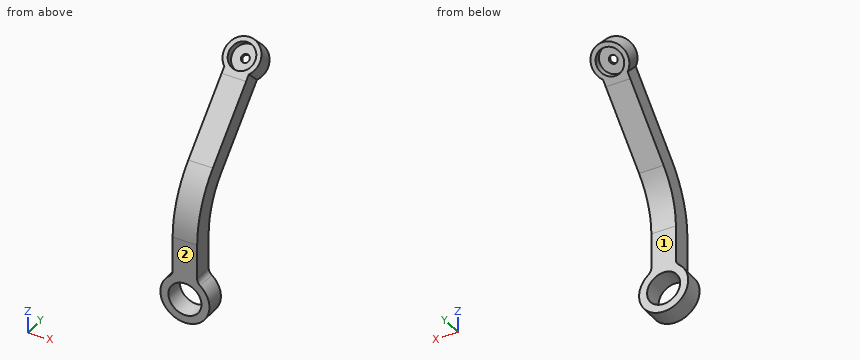
Autodesk Inventor part; units mm, degrees
ref_plane "Work Plane11" through (7.5, 8.6447, 72.635) normal (0, 0.7071, -0.7071) x (-1, 0, 0)
ref_plane "YZ Plane" through (0, 0, 0) normal (1, 0, 0) x (0, 1, 0)
ref_plane "XZ Plane" through (0, 0, 0) normal (0, 1, 0) x (-1, 0, 0)
sketch "Sketch1" plane through (0, 0, 0) normal (0, 1, 0) x (-1, 0, 0)
  arc A0 (-9.375, 11.7094) -> (9.375, 11.7094) centre (0, 0) ccw
  line L0 (-7.5, 15.6125) -> (-7.5, 22.9904)
  line L1 (7.5, 22.9904) -> (7.5, 15.6125)
  line L2 (7.5, 22.9904) -> (-7.5, 22.9904)
  arc A1 (7.5, 15.6125) -> (9.375, 11.7094) centre (12.5, 15.6125) ccw
  arc A2 (-9.375, 11.7094) -> (-7.5, 15.6125) centre (-12.5, 15.6125) ccw
  point P0 (7.5, 12.9904)
  point P1 (-7.5, 12.9904)
  point P2 (0, 12.9904)
  point P3 (0, 22.9904)
  dimension "d0" = 30
  dimension "d109" = 5
  dimension "d129" = 15
  dimension "d131" = 10
  dimension "d132" = 12.9904
extrude "Extrusion1" add sketch "Sketch1" against normal blind 12
sketch "Sketch22" plane through (-7.5, 0, 22.9904) normal (0, 0, 1) x (1, 0, 0)
  line L0 (0, 0) -> (0, -12)
  line L1 (15, -12) -> (0, -12)
  line L2 (0, 0) -> (15, 0)
  line L3 (15, 0) -> (15, -12)
  line L4 (15, -12) -> (0, -12)
  line L5 (0, -12) -> (0, 0)
  point P0 (7.5, 0)
sketch "Sketch23" plane through (0, 0, 0) normal (1, 0, 0) x (0, 1, 0)
  line L0 (0, 22.9904) -> (-12, 22.9904)
  line L1 (-6, 22.9904) -> (-6, 37.2797)
  line L2 (8.6447, 72.635) -> (43.4975, 107.4879)
  arc A0 (8.6447, 72.635) -> (-6, 37.2797) centre (44, 37.2797) ccw
  point P0 (0, 0)
  point P1 (-6, 57.9904)
  dimension "d110" = 35
  dimension "d111" = 70
  dimension "d112" = 135
  dimension "d113" = 50
sweep "Sweep2" add profiles "Sketch22" path "Sketch23" path curves L1 A0 L2
ref_plane "Work Plane11" through (7.5, 8.6447, 72.635) normal (0, 0.7071, -0.7071) x (-1, 0, 0)
sketch "Sketch24" plane through (7.5, 8.6447, 72.635) normal (0, 0.7071, -0.7071) x (-1, 0, 0)
  line L0 (0, 49.2893) -> (15, 49.2893)
  line L1 (0, 49.2893) -> (15, 49.2893)
  line L2 (0, 49.2893) -> (0, 53.2426)
  line L3 (15, 49.2893) -> (15, 53.2426)
  arc A0 (15, 53.2426) -> (0, 53.2426) centre (7.5, 61.2893) ccw
  line L4 (0, 49.2893) -> (15, 49.2893)
  point P0 (7.5, -57.4734)
  point P1 (7.5, 49.2893)
  point P2 (7.5, 49.2893)
  dimension "d136" = 22
  dimension "d137" = 12
extrude "Extrusion17" add sketch "Sketch24" along normal mid plane 12
sketch "Sketch25" plane through (-7.5, 4.402, 76.8777) normal (0, -0.7071, 0.7071) x (1, 0, 0)
  arc A0 (15, 53.2426) -> (0, 53.2426) centre (7.5, 61.2893) ccw
  circle A1 centre (7.5, 61.2893) radius 2.5
  point P0 (7.5, -57.4734)
  dimension "d138" = 5
extrude "Extrusion18" cut sketch "Sketch25" against normal through all
sketch "Sketch26" plane through (0, -12, 0) normal (0, -1, 0) x (1, 0, 0)
  circle A0 centre (0, 0) radius 10.1
  dimension "d133" = 20.2
extrude "Extrusion19" cut sketch "Sketch26" against normal through all
sketch "Sketch27" plane through (7.5, 12.8873, 68.3924) normal (0, 0.7071, -0.7071) x (-1, 0, 0)
  circle A0 centre (7.5, 61.2893) radius 2.5
  circle A1 centre (7.5, 61.2893) radius 8.1
  point P0 (7.5, -57.4734)
  dimension "d139" = 16.2
extrude "Extrusion20" cut sketch "Sketch27" against normal blind 5
mirror "Mirror2" about plane through (7.5, 8.6447, 72.635) normal (0, 0.7071, -0.7071) of "Extrusion20"
properties part number "proximal_link_2"
Can you work these out from the model? Positions are in its coordinate system, mm. Face numbers are marked on the shaded views. A direction names the side the tool comes from. Coordinates: 2 decimals unless noted, no trailing zeros. Write each loop counter-clockwise with the first axis right and the second up, starting at its lowest first coordinate (ties: lowest second). Pieces come first, ordered by that corner, then holes. Notation, with made-up numbers: (-8.5, -5.5) -> (35.5, -5.5) arc R20 cw to (35.5, 12.5) -> close; hole circle Ø3 at (4.5, 25). An arc over 180 degrees is marked (long way). Write each question's results on one line, items separated by ' | '. Start each with the question number.
Q1. Imagine slicing it at D-D (y = 20.5). Write out the boundary of the cut face in (x, z), then the cut area to 3 significant figures.
Q2. If I drill on probe 1 along X at (y, z) = (-1.5, 48.5); probe 2 along Z at (x, y) = (0, -3.5); probe 3 along Z at (x, y) = (-3, -4.5), over which ranges is the centre line in solid material (lowest first)?
Q3. I'm going to push flat-ended pins straight in: pin 1 (2 mm diameter, centred on x = 8, z = 32.5, fed in from +Y); pin 2 (1.5 mm diameter, centred on x = -2.5, y = 51.5, fed in from -Z) (3 decimals); pin 3 (12 mm diameter, centred on x = -4, y = 23, fed in from +Z). Where does each tip first touch, or does it pass through?
Q4. Imagine slicing it at A-A (z = 0). Write out the boundary of the cut face in (x, y), then the cut area to 3 significant figures.
Q5. On a 3-axis mill with a long thin cutter (end or side, diameter ignored), from which of +Z, -Z, +X, -X, +Y, -Y can I reach the whole of each face in a straight line? I mean the marked faces 1 and 2. Say none if no direction works.
Q6. Imagine slicing it at C-C (z = 17). Write out the boundary of the cut face in (x, y), then the cut area to 3 significant figures.
Taken from the geometry:
1) outline: (-7.5, 76.01) -> (7.5, 76.01) -> (7.5, 92.98) -> (-7.5, 92.98) -> close | area: 255 mm^2
2) probe 1: x = -7.5 to 7.5 | probe 2: z = -15 to -10.1, 10.1 to 66.94 | probe 3: z = -14.7 to -9.64, 9.64 to 65.28
3) pin 1: stops at y = 0 | pin 2: stops at z = 106.255 | pin 3: stops at z = 101.48
4) outline: (-15, -12) -> (-10.1, -12) -> (-10.1, 0) -> (-15, 0) -> close; (10.1, -12) -> (15, -12) -> (15, 0) -> (10.1, 0) -> close | area: 118 mm^2
5) face 1: -Z, +X, -X, +Y | face 2: +Z, -Z, +X, -X, -Y
6) outline: (-7.5, -12) -> (7.5, -12) -> (7.5, 0) -> (-7.5, 0) -> close | area: 180 mm^2
